```python
from build123d import *

# Parameters (mm, degrees)
F0_R      = 3.5
F1_DEPTH  = 3.2
F1_TAPER  = 15
F2_R      = 3
F3_DEPTH  = 0.3
F4_SIZE   = 0.2
F5_R      = 2.5
F6_DEPTH  = 5
F6_TAPER  = 8
F7_R      = 2.2
F8_DEPTH  = 0.3
F9_R      = 1.75
F10_DEPTH = 3.2
F11_R     = 2.5
F12_DEPTH = 0.2
F13_R     = 1
F14_DEPTH = 2
F15_SIZE  = 0.1
F16_R     = 3
F17_DEPTH = 11.74
F17_TAPER = 10


with BuildPart() as f1:
    # F0 (on Front) → F1 (new body)
    with BuildSketch(Plane.XZ):
        Circle(F0_R)
    extrude(amount=F1_DEPTH, taper=F1_TAPER)

    # F2 (on face) → F3 (join)
    with BuildSketch(Plane.XZ.offset(3.2)):
        Circle(F2_R)
    extrude(amount=F3_DEPTH)

    # F4
    f4_edges = [f1.edges().sort_by_distance(p)[0] for p in [
        (-3.5, 0, 0),
    ]]
    chamfer(f4_edges, length=F4_SIZE)

    # F5 (on face) → F6 (join)
    with BuildSketch(Plane.XZ.offset(3.5)):
        Circle(F5_R)
    extrude(amount=F6_DEPTH, taper=F6_TAPER)

    # F7 (on face) → F8 (join)
    with BuildSketch(Plane.XZ.offset(8.5)):
        Circle(F7_R)
    extrude(amount=F8_DEPTH)

    # F9 (on face) → F10 (join)
    with BuildSketch(Plane.XZ.offset(8.8)):
        Circle(F9_R)
    extrude(amount=F10_DEPTH)

    # F11 (on face) → F12 (join)
    with BuildSketch(Plane.XZ.offset(12)):
        Circle(F11_R)
    extrude(amount=F12_DEPTH)

    # F13 (on face) → F14 (join)
    with BuildSketch(Plane.XZ.offset(12.2)):
        Circle(F13_R)
    extrude(amount=F14_DEPTH)

    # F15
    f15_edges = [f1.edges().sort_by_distance(p)[0] for p in [
        (-3, -3.5, 0),
        (-2.2, -8.8, 0),
        (-2.2, -8.5, 0),
        (-3, -3.2, 0),
    ]]
    chamfer(f15_edges, length=F15_SIZE)

    # F16 (on face) → F17 (cut, symmetric)
    with BuildSketch(Plane(origin=(0, 0, 0), x_dir=(-1, 0, 0), z_dir=(0, 1, 0))):
        Circle(F16_R)
    extrude(amount=F17_DEPTH, both=True, taper=F17_TAPER, mode=Mode.SUBTRACT)


solid = f1.part
```
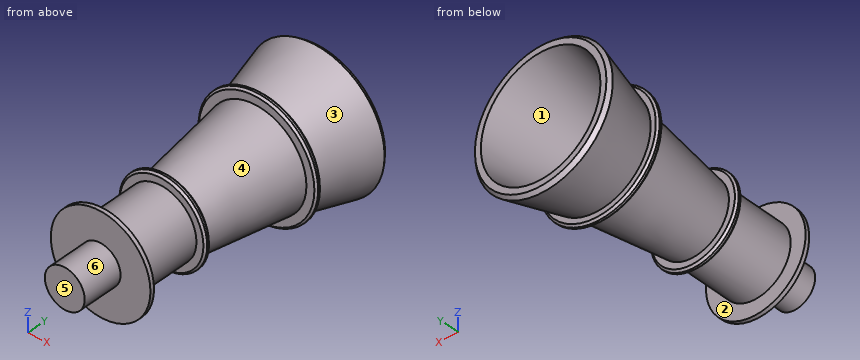
Can you work these out from the model? Positions are in its coordinate system, mm. Face numbers are marked on the shaded views. A direction names the side the tool comes from. Round coordinates to 2 decimals unless told otherwise and drop trailing zeros. Loops run counter-clockwise (first coordinate to the right, second up) from the corner with the lowest first, then second, coordinate; pieces in that order, holes last. Notation, with made-up numbers: (56, -4) -> (90, -4) arc R27 ccw to (90, 20) -> close; hole circle Ø10 at (-18, 10). An arc over 180 degrees is marked (long way). One line per item, written item: value. Start each with the question number.
1. If we mould it in two halves opening along Z, with no side actions, what happens to the marked faces 1, 2 and 3? For each: pulls with the +Z half, pulls with the -Z half, needs draft (parallel to the pull), parting line crosses it, or undercut.
2. For pin 1 (4 mm diameter, centred on x = -0.5, y = -2.5, fed in from -Z); pin 2 (0.6 mm diameter, centred on x = 0, z = 0, fed in from +Y); pin 3 (2 mm diameter, centred on y = -5, z = -0.5, fed in from -X); pin 4 (1 mm diameter, centred on y = -10.5, z = -2.5, fed in from +X), each with a flat end and sliding along its axis, tell me the tip position at first contact or that it passes through.
3. For the marked faces 4, 5 and 6, which set-ups out of +Z, -Z, +X, -X, +Y, -Y let a thin tool reach every point of the face, with its end or its side?
4. If we section it at B-B, the plane y = -6: Write out the boundary of the cut face in (x, z), then the cut area to 3 significant figures.
5. If we section it at A-A, the plane y = -9.75: Write out the boundary of the cut face in (x, z).
6. If I drill on probe 1 along Z at (x, y) = (-0.75, -0.75); probe 2 along Z at (x, y) = (-1.75, -5.5); probe 3 along Y at (x, z) = (0.5, 0.5), over which ranges is the centre line in solid material (lowest first)?
Calculated:
1. face 1: undercut
1. face 2: needs draft
1. face 3: parting line crosses it
2. pin 1: stops at z = -3.35
2. pin 2: stops at y = -11.74
2. pin 3: stops at x = -2.42
2. pin 4: passes through
3. face 4: none
3. face 5: +Z, -Z, +X, -X, -Y
3. face 6: -Y
4. outline: circle Ø4.3 at (0, 0); hole circle Ø3.88 at (0, 0)
4. area: 2.66 mm²
5. outline: circle Ø3.5 at (0, 0); hole circle Ø2.56 at (0, 0)
6. probe 1: z = -3.21 to -2.77, 2.77 to 3.21
6. probe 2: z = -1.36 to -1.03, 1.03 to 1.36
6. probe 3: y = -14.2 to -11.74
